The listing builds one solid part. Answer for the finished solid, in the listing's coordinates (mm). Round coordinates to 2 decimals unless told otherwise and drop trailing zeros. Loops run counter-clockwise (first coordinate to the right, second up) from the corner with the lowest first, then second, coordinate; pieces in that order, holes last. Notation, with made-up numbers: M -1,89 L 42,89 A6 cw 42,99 Z; hole C -25,36.5 d5. An arc over 180 degrees is marked long. Answer as a JSON object with one key per item and string values.
```python
from build123d import *

# Parameters (mm, degrees)
SKETCH_1_W            = 52
SKETCH_1_H            = 46
SKETCH_1_R            = 2.6
SKETCH_1_R_2          = 4.15
EXTRUDE_436_DEPTH     = 4
SKETCH_4_R            = 2.1
CUT_EXTRUDE_686_DEPTH = 5
SKETCH_6_R            = 2.1
EXTRUDE_1_DEPTH       = 4
SKETCH_7_R            = 1.2
CUT_EXTRUDE_1_DEPTH   = 5
SKETCH_8_W            = 29.384652785
SKETCH_8_H            = 46
EXTRUDE_2_DEPTH       = 4
FILLET_1_R            = 5
SKETCH_9_R            = 1.6
CUT_EXTRUDE_2_DEPTH   = 5


with BuildPart() as part:
    # 草图1 → Extrude 436 (new body)
    with BuildSketch(Plane(origin=(0, 0, 0), x_dir=(1, 0, 0), z_dir=(0, 1, 0))):
        Rectangle(SKETCH_1_W, SKETCH_1_H)
        with Locations((-18.25, 0)):
            Circle(SKETCH_1_R, mode=Mode.SUBTRACT)
        with Locations((18.25, 0)):
            Circle(SKETCH_1_R, mode=Mode.SUBTRACT)
        Circle(SKETCH_1_R_2, mode=Mode.SUBTRACT)
    extrude(amount=EXTRUDE_436_DEPTH)

    # 草图4 → Cut-Extrude 686 (cut, through all)
    with BuildSketch(Plane(origin=(0, 4, 0), x_dir=(1, 0, 0), z_dir=(0, 1, 0))):
        with Locations((-12, 18)):
            Circle(SKETCH_4_R)
        with Locations((12, 18)):
            Circle(SKETCH_4_R)
        with Locations((12, -18)):
            Circle(SKETCH_4_R)
        with Locations((-12, -18)):
            Circle(SKETCH_4_R)
    extrude(amount=-CUT_EXTRUDE_686_DEPTH, mode=Mode.SUBTRACT)

    # 草图6 → 凸台-拉伸1 (add)
    with BuildSketch(Plane(origin=(0, 4, 0), x_dir=(1, 0, 0), z_dir=(0, 1, 0))):
        with Locations((-12, -18)):
            Circle(SKETCH_6_R)
        with Locations((12, -18)):
            Circle(SKETCH_6_R)
    extrude(amount=-EXTRUDE_1_DEPTH)

    # 草图7 → 切除-拉伸1 (cut, through all)
    with BuildSketch(Plane(origin=(0, 4, 0), x_dir=(1, 0, 0), z_dir=(0, 1, 0))):
        with Locations((5, -20)):
            Circle(SKETCH_7_R)
        with Locations((-15, -20)):
            Circle(SKETCH_7_R)
    extrude(amount=-CUT_EXTRUDE_1_DEPTH, mode=Mode.SUBTRACT)

    # 草图8 → 凸台-拉伸2 (add)
    with BuildSketch(Plane.XZ):
        with Locations((40.692326393, 0)):
            Rectangle(SKETCH_8_W, SKETCH_8_H)
    extrude(amount=-EXTRUDE_2_DEPTH)

    # 圆角1
    fillet_1_edges = [part.edges().sort_by_distance(p)[0] for p in [
        (55.384652785, 2, 23),
        (55.384652785, 2, -23),
        (-26, 2, 23),
        (-26, 2, -23),
    ]]
    fillet(fillet_1_edges, radius=FILLET_1_R)

    # 草图9 → 切除-拉伸2 (cut, through all)
    with BuildSketch(Plane.XZ):
        with Locations((-15, 20)):
            Circle(SKETCH_9_R)
        with Locations((5, 20)):
            Circle(SKETCH_9_R)
        with Locations((25.4, 20)):
            Circle(SKETCH_9_R)
        with Locations((45.4, 20)):
            Circle(SKETCH_9_R)
    extrude(amount=-CUT_EXTRUDE_2_DEPTH, mode=Mode.SUBTRACT)


solid = part.part
```
Item 1: Determine the mould class of faces 1 (the face through (-24, 2, -22)), 2 (the face through (11.727, 2.028, -20.082)), 3 (the face through (55.385, 2, 0)) for opening direction Z: released by +Z, released by -Z, zero draft, split by the parting line, or undercut.
Values follow:
{"face 1": "released by -Z", "face 2": "undercut", "face 3": "zero draft"}
Item 2: The part is cut by section B-B (y = 0.75). Give the number of separate pieces and of enclosed holes in the cut face, then the cut area to 3 significant figures.
Values follow:
{"separate pieces": "1", "enclosed holes": "9", "area": "3,570 mm^2"}
Item 3: The part is cut by section A-A (x = 25.4). Give the vertices of the cut face in (y, z).
Values follow:
{"outline": "M 0,-23 L 4,-23 L 4,18.4 L 0,18.4 Z; M 0,21.6 L 4,21.6 L 4,23 L 0,23 Z"}
Item 4: A flat-ended cylindrical pin translates along its axis: P1, Ø5.5, axis at x = -12, z = -18, coming from the +Y side. Find the tip coordinate at first contact, or state that the pin passes through.
Values follow:
{"P1": "y = 4"}
Item 5: Straight lines are drawn through the part: line 1 (X direction, y = 3.2, z = 0); line 2 (X direction, y = 2.25, z = -1.5); line 3 (Z direction, x = 18.25, y = 1.9). For each, find the intervals that lie inside material, in ascending order.
Values follow:
{"line 1": "-26 to -20.85, -15.65 to -4.15, 4.15 to 15.65, 20.85 to 55.38", "line 2": "-26 to -20.37, -16.13 to -3.87, 3.87 to 16.13, 20.37 to 55.38", "line 3": "-23 to -2.6, 2.6 to 23"}
Item 6: The part is cut by section C-C (x = 12). Give the vertices of the cut face in (y, z), then the cut area to 3 significant figures.
Values follow:
{"outline": "M 0,-23 L 4,-23 L 4,-20.1 L 0,-20.1 Z; M 0,-15.9 L 4,-15.9 L 4,23 L 0,23 Z", "area": "167 mm^2"}
